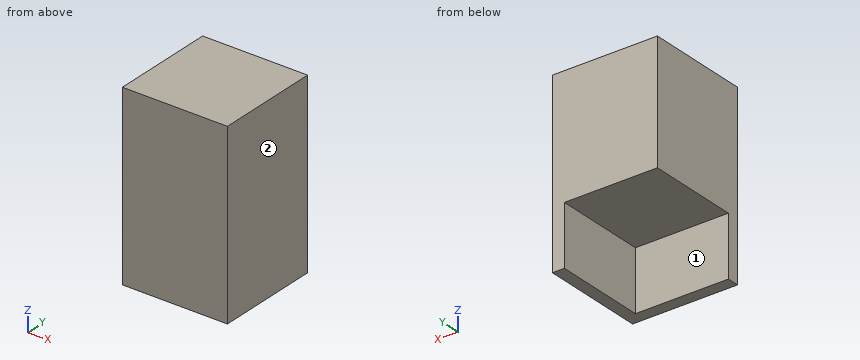
```python
from build123d import *

# Parameters (mm, degrees)
CROQUIS1_W              = 35
CROQUIS1_H              = 35
SALIENTE_EXTRUIR1_DEPTH = 40
SALIENTE_EXTRUIR3_DEPTH = 20


with BuildPart() as part:
    # Croquis1 → Saliente-Extruir1 (new body)
    with BuildSketch(Plane.XY):
        Rectangle(CROQUIS1_W, CROQUIS1_H)
    extrude(amount=SALIENTE_EXTRUIR1_DEPTH)

    # Croquis4 → Saliente-Extruir3 (add)
    with BuildSketch(Plane(origin=(0, 0, 0), x_dir=(-1, 0, 0), z_dir=(0, 0, -1))):
        Polygon((-13.5, 13.5), (-13.5, 17.5), (-17.5, 17.5), (-17.5, -17.5), (17.5, -17.5), (17.5, -13.5), (13.5, -13.5), (-13.5, -13.5), align=None)
    extrude(amount=SALIENTE_EXTRUIR3_DEPTH)


solid = part.part
```
Input: part model. Units: mm. Frame: model coordinates. Face numbers are marked on the shaded views. A direction names the side the tool comes from. Give positions to 0.01 mm unless a question says otherwise; leave off trailing zeros. Order: outer loops, then holes, each group sorted by start corner. A loop starts at its lowest first (then second) coordinate and runs counter-clockwise, first axis right, second up.
1. Reachability of the marked faces 1 and 2 from +Z, -Z, +X, -X, +Y, -Y: full face, straight path, thin tool, end or side. Return the list, or none.
Derived:
face 1: -Z, -X, +Y
face 2: +Z, -Z, +X, +Y, -Y
2. Section B-B on z = -15. Return the cut outline in (x, y), and give its area (3 significant figures).
Derived:
outline: (-17.5, -17.5) - (17.5, -17.5) - (17.5, 17.5) - (13.5, 17.5) - (13.5, -13.5) - (-17.5, -13.5) - close
area: 264 mm2
3. Material intervals for L1, parallel to Y at x = 2, z = -17; L2, parallel to Z at x = -12.5, y = 15; L3, parallel to X at y = -5, z = -18, sorted ascending.
Derived:
L1: y = -17.5 to -13.5
L2: z = 0 to 40
L3: x = 13.5 to 17.5
4. Section A-A on x = 12. Return the cut outline in (y, z), and give its area (3 significant figures).
Derived:
outline: (-17.5, -20) - (-13.5, -20) - (-13.5, 0) - (17.5, 0) - (17.5, 40) - (-17.5, 40) - close
area: 1,480 mm2
5. Pin query (flat end, axial travel): pin 1 (6 mm diameter, centred on x = 7.5, z = -13, fed in from +Y). Return the tip coordinate at first contact, or that it passes through.
Derived:
pin 1: stops at y = -13.5
